```python
from build123d import *

# Parameters (mm, degrees)
F1_DEPTH = 2


with BuildPart() as f1:
    # F0 (on Front) → F1 (new body)
    with BuildSketch(Plane.XZ):
        Polygon((-112.1402904391, 33.0038927495), (207.8597095609, 33.0038927495), (207.8597095609, 332.3038927495), (207.8597095609, 333.0038927495), (167.8597095609, 333.0038927495), (-112.1402904391, 73.0038927495), align=None)
        with BuildLine():
            Line((101.2039725726, 88.4770882584), (101.6136759777, 69.7171021446))
            Line((101.6136759777, 69.7171021446), (90.5410552282, 69.7171021446))
            Line((90.5410552282, 69.7171021446), (90.5410552282, 105.1249880537))
            Line((90.5410552282, 105.1249880537), (101.1704111356, 105.1249880537))
            Line((101.1704111356, 105.1249880537), (101.1704111356, 99.2129225477))
            ThreePointArc((101.1704111356, 99.2129225477), (106.2318508757, 104.4981198242), (113.4292611737, 105.8205295548))
            Line((113.4292611737, 105.8205295548), (113.4292611737, 95.8221633181))
            ThreePointArc((113.4292611737, 95.8221633181), (105.6893165245, 94.8581367621), (101.2039725726, 88.4770882584))
        make_face(mode=Mode.SUBTRACT)
        with BuildLine():
            Line((127.6888195951, 88.4937142061), (128.0985230001, 69.7337280923))
            Line((128.0985230001, 69.7337280923), (117.0259022507, 69.7337280923))
            Line((117.0259022507, 69.7337280923), (117.0259022507, 105.1416140014))
            Line((117.0259022507, 105.1416140014), (127.6552581581, 105.1416140014))
            Line((127.6552581581, 105.1416140014), (127.6552581581, 99.2295484954))
            ThreePointArc((127.6552581581, 99.2295484954), (132.7166978981, 104.5147457719), (139.9141081962, 105.8371555025))
            Line((139.9141081962, 105.8371555025), (139.9141081962, 95.8387892658))
            ThreePointArc((139.9141081962, 95.8387892658), (132.1741635469, 94.8747627098), (127.6888195951, 88.4937142061))
        make_face(mode=Mode.SUBTRACT)
        with BuildLine():
            add(Edge.make_bspline(
                [(166.1158787618, 92.7830700848), (164.5692102089, 91.5353198263), (160.8559417387, 91.0074140824), (147.0308134747, 89.8356227603), (141.5287422164, 79.8600298922), (145.6215095019, 69.4638702682), (159.8163332075, 68.0542730887), (163.3323899676, 71.0322612124), (166.1158787618, 72.4894021723)],
                knots=[0, 0, 0, 0, 0.1282549597, 0.3235779421, 0.4933166916, 0.6588260023, 0.8480719548, 1, 1, 1, 1], degree=3))
            Line((166.1158787618, 92.7830700848), (166.1158787618, 86.1217890952))
            add(Edge.make_bspline(
                [(166.1158787618, 80.1576142285), (165.648079511, 78.8716732666), (164.7089985438, 76.1838402752), (159.2900957109, 75.3320101397), (154.3144147308, 76.3842047893), (154.1488989038, 82.6667071186), (159.3286899056, 84.8140545113), (163.2298071329, 85.1164060676), (166.1158787618, 86.1217890952)],
                knots=[0, 0, 0, 0, 0.1467139352, 0.3148344078, 0.4723324727, 0.6349882053, 0.7976765175, 1, 1, 1, 1], degree=3))
            Line((166.1158787618, 80.1576142285), (166.1158787618, 72.4894021723))
        make_face(mode=Mode.SUBTRACT)
        with BuildLine():
            ThreePointArc((144.5925937182, 94.4093083117), (148.8127137387, 102.502604489), (157.3532582577, 105.7228459891))
            Line((157.3532582577, 105.7228459891), (166.1158787618, 105.6858685351))
            Line((166.1158787618, 105.6858685351), (166.1158787618, 96.8470781765))
            ThreePointArc((166.1158787618, 96.8470781765), (159.8763121864, 98.9559091904), (155.2180157191, 94.2997698758))
            Line((155.2180157191, 94.2997698758), (144.5925937182, 94.4093083117))
        make_face(mode=Mode.SUBTRACT)
        with BuildLine():
            ThreePointArc((90.7690819051, 154.6215500374), (97.4783010599, 153.7198410632), (102.8321381356, 149.5770003338))
            Line((102.8321381356, 149.5770003338), (102.8321381356, 154.1828896542))
            Line((102.8321381356, 154.1828896542), (113.140575185, 154.1828896542))
            Line((113.140575185, 154.1828896542), (113.140575185, 109.6980508108))
            Line((113.140575185, 109.6980508108), (102.8321381356, 109.6980508108))
            Line((102.8321381356, 109.6980508108), (102.8321381356, 122.1266548772))
            ThreePointArc((102.8321381356, 122.1266548772), (97.2685141585, 118.2745070428), (90.5424948479, 117.5304513116))
            Line((90.5424948479, 117.5304513116), (90.5424948479, 128.526845171))
            ThreePointArc((90.5424948479, 128.526845171), (96.3918627119, 126.17333299), (101.6822974827, 129.6034093638))
            ThreePointArc((101.6822974827, 129.6034093638), (103.1910724549, 136.3586272736), (101.6822974827, 143.1138451834))
            ThreePointArc((101.6822974827, 143.1138451834), (96.1363497819, 146.3446188485), (90.5904020812, 143.1138451834))
            Line((90.5904020812, 143.1138451834), (90.7690819051, 154.6215500374))
        make_face(mode=Mode.SUBTRACT)
        with BuildLine():
            Line((129.2334676245, 135.4241105345), (128.8237642195, 154.1840966483))
            Line((128.8237642195, 154.1840966483), (139.8963849689, 154.1840966483))
            Line((139.8963849689, 154.1840966483), (139.8963849689, 118.7762107392))
            Line((139.8963849689, 118.7762107392), (129.2670290615, 118.7762107392))
            Line((129.2670290615, 118.7762107392), (129.2670290615, 124.6882762452))
            ThreePointArc((129.2670290615, 124.6882762452), (124.2055893215, 119.4030789686), (117.0081790234, 118.0806692381))
            Line((117.0081790234, 118.0806692381), (117.0081790234, 128.0790354748))
            ThreePointArc((117.0081790234, 128.0790354748), (124.7481236727, 129.0430620307), (129.2334676245, 135.4241105345))
        make_face(mode=Mode.SUBTRACT)
        with BuildLine():
            add(Edge.make_bspline(
                [(166.0185557871, 141.4059485932), (164.4718872342, 140.1581983347), (160.7586187641, 139.6302925908), (146.9334905, 138.4585012686), (141.4314192417, 128.4829084005), (145.5241865272, 118.0867487766), (159.7190102328, 116.6771515971), (163.2350669929, 119.6551397208), (166.0185557871, 121.1122806807)],
                knots=[0, 0, 0, 0, 0.1282549597, 0.3235779421, 0.4933166916, 0.6588260023, 0.8480719548, 1, 1, 1, 1], degree=3))
            Line((166.0185557871, 141.4059485932), (166.0185557871, 134.7446676035))
            add(Edge.make_bspline(
                [(166.0185557871, 128.7804927369), (165.5507565363, 127.4945517749), (164.6116755691, 124.8067187836), (159.1927727362, 123.9548886481), (154.2170917561, 125.0070832977), (154.0515759291, 131.2895856269), (159.231366931, 133.4369330196), (163.1324841582, 133.739284576), (166.0185557871, 134.7446676035)],
                knots=[0, 0, 0, 0, 0.1467139352, 0.3148344078, 0.4723324727, 0.6349882053, 0.7976765175, 1, 1, 1, 1], degree=3))
            Line((166.0185557871, 128.7804927369), (166.0185557871, 121.1122806807))
        make_face(mode=Mode.SUBTRACT)
        with BuildLine():
            ThreePointArc((144.4952707435, 143.0321868201), (148.715390764, 151.1254829974), (157.255935283, 154.3457244975))
            Line((157.255935283, 154.3457244975), (166.0185557871, 154.3087470435))
            Line((166.0185557871, 154.3087470435), (166.0185557871, 145.4699566849))
            ThreePointArc((166.0185557871, 145.4699566849), (159.7789892117, 147.5787876987), (155.1206927444, 142.9226483841))
            Line((155.1206927444, 142.9226483841), (144.4952707435, 143.0321868201))
        make_face(mode=Mode.SUBTRACT)
    extrude(amount=F1_DEPTH)


solid = f1.part
```
Geometry check sheet. Reference: the model listing, model coordinates, mm. A direction names the side the tool comes from. Give positions to 0.01 mm unless a question says otherwise; leave off trailing zeros. Order: outer loops, then holes, each group sorted by start corner. A loop starts at its lowest first (then second) coordinate and runs counter-clockwise, first axis right, second up. Notation, with made-up numbers: (23, 82) - (72, 82) arc R31 ccw to (72, 106) - close; hole circle Ø9 at (85.5, 16.25). An arc over 180 degrees is marked (long way). Answer in a Markdown table with one row per item. Add a question column.
Q1. Material ranges on probe 1 along Z at (x, y) = (91.5, -0.4); probe 2 along X at (y, z) = (-0.4, 71); probe 3 along X at (y, z) = (-0.65, 271.5), recorded low to high. Write a range as from..to.
Q2. Cross-section at C-C, the plane z = 205. Enter the section's corners in (x, y).
Q3. Mould release check, pull along Z, two halves, no side actions. Record for faces 1 (the flat face through (81, 0, 152)), 2 (the cylindrical face through (148.7, -1, 102.4)), 3 (the flat face through (29.82, -0.986, 204.824)): pulls with the +Z half, pulls with the -Z half, needs draft (parallel to the pull), parting line crosses it, or undercut.
Q4. Cross-section at A-A, the plane y = -0.85. Count the separate pieces of the cut face and the enclosed holes in it, then the cut area to 3 significant figures.
Q5. Tool access check on faces 4 (the flat face through (81, -2, 152)), 5 (the cylindrical face through (106.14, -0.99, 104.45)). Record the directions out of +Z, -Z, +X, -X, +Y, -Y that give a thin tool (end or side, any length) a straight path to the whole face; none if there is none.
Q6. Cross-section at D-D, the plane x = 29. Enter the section's corners in (y, z), then the cut area to 3 significant figures.
Q7. Gauge pin test, flat ends, axial feed: pin 1 (1 mm diameter, centred on x = 122.5, y = -0.5, fed in from +Z); pin 2 (1 mm diameter, centred on y = -0.5, z = 75, fed in from -X); pin 3 (1 mm diameter, centred on x = 135.5, y = -0.5, fed in from +Z). Record the tip position at first contact, or that the pin passes through.
Check values:
| question | item | result |
|---|---|---|
| 1 | probe 1 | z = 33..69.72, 105.12..117.43, 127.61..144.35, 154.7..262.1 |
| 1 | probe 2 | x = -112.14..90.54, 101.59..117.03, 128.07..147.38, 163.48..207.86 |
| 1 | probe 3 | x = 101.62..207.86 |
| 2 | outline | (30.01, -2) - (207.86, -2) - (207.86, 0) - (30.01, 0) - close |
| 3 | face 1 | needs draft |
| 3 | face 2 | undercut |
| 3 | face 3 | pulls with the +Z half |
| 4 | separate pieces | 1 |
| 4 | enclosed holes | 8 |
| 4 | area | 56,400 mm^2 |
| 5 | face 4 | +Z, -Z, +X, -X, -Y |
| 5 | face 5 | +Y, -Y |
| 6 | outline | (-2, 33) - (0, 33) - (0, 204.06) - (-2, 204.06) - close |
| 6 | area | 342 mm^2 |
| 7 | pin 1 | stops at z = 291.35 |
| 7 | pin 2 | stops at x = -110.53 |
| 7 | pin 3 | stops at z = 303.42 |
